Design review of the part built by this model. Coordinates are the model's own, in mm. A direction names the side the tool comes from. Coordinates: 2 decimals unless noted, no trailing zeros. Loops run counter-clockwise (first coordinate to the right, second up) from the corner with the lowest first, then second, coordinate; pieces in that order, holes last. Notation, with made-up numbers: (-31, 34.25) -> (-8, 34.25) arc R19 cw to (-8, 43.25) -> close; hole circle Ø2 at (29, 15). An arc over 180 degrees is marked (long way). Answer in a Markdown table with one row per item.
```python
from build123d import *

# Parameters (mm, degrees)
BOSS_EXTRUDE2_DEPTH = 30
CUT_EXTRUDE3_DEPTH  = 28
SKETCH10_W          = 9
SKETCH10_H          = 11
CUT_EXTRUDE4_DEPTH  = 3


with BuildPart() as part:
    # Sketch2 → Boss-Extrude2 (new body)
    with BuildSketch(Plane.XY):
        with BuildLine():
            Line((-28.917214192, 20.79500657), (39.082785808, 20.79500657))
            ThreePointArc((39.082785808, 20.79500657), (41.204106152, 19.916326914), (42.082785808, 17.79500657))
            Line((42.082785808, 17.79500657), (42.082785808, -56.20499343))
            ThreePointArc((42.082785808, -56.20499343), (41.204106152, -58.326313773), (39.082785808, -59.20499343))
            Line((39.082785808, -59.20499343), (-28.917214192, -59.20499343))
            ThreePointArc((-28.917214192, -59.20499343), (-31.038534535, -58.326313773), (-31.917214192, -56.20499343))
            Line((-31.917214192, -56.20499343), (-31.917214192, 17.79500657))
            ThreePointArc((-31.917214192, 17.79500657), (-31.038534535, 19.916326914), (-28.917214192, 20.79500657))
        make_face()
    extrude(amount=BOSS_EXTRUDE2_DEPTH)

    # Sketch7 → Cut-Extrude3 (cut)
    with BuildSketch(Plane.XY.offset(30)):
        with BuildLine():
            Line((-28.917214192, -57.20499343), (39.082785808, -57.20499343))
            ThreePointArc((39.082785808, -57.20499343), (39.789892589, -56.912100211), (40.082785808, -56.20499343))
            Line((40.082785808, -56.20499343), (40.082785808, 17.79500657))
            ThreePointArc((40.082785808, 17.79500657), (39.789892589, 18.502113351), (39.082785808, 18.79500657))
            Line((39.082785808, 18.79500657), (-28.917214192, 18.79500657))
            ThreePointArc((-28.917214192, 18.79500657), (-29.624320973, 18.502113351), (-29.917214192, 17.79500657))
            Line((-29.917214192, 17.79500657), (-29.917214192, -56.20499343))
            ThreePointArc((-29.917214192, -56.20499343), (-29.624320973, -56.912100211), (-28.917214192, -57.20499343))
        make_face()
    extrude(amount=-CUT_EXTRUDE3_DEPTH, mode=Mode.SUBTRACT)

    # Sketch10 → Cut-Extrude4 (cut)
    with BuildSketch(Plane.XZ.offset(59.20499343)):
        Polygon((-12, 11.6), (-9.001867248, 14.598132752), (-3.001867248, 14.598132752), (0, 11.603739153), (0, 3.6), (-12, 3.6), align=None)
        with Locations((21, 9.1)):
            Rectangle(SKETCH10_W, SKETCH10_H)
    extrude(amount=-CUT_EXTRUDE4_DEPTH, mode=Mode.SUBTRACT)


solid = part.part
```
(1) For pin 1 (0.6 mm diameter, centred on y = -58.5, z = 8, fed in from -X); pin 2 (1 mm diameter, centred on y = -58.5, z = 9, fed in from +X); pin 3 (2 mm diameter, centred on x = 31, y = 12, fed in from +Z), all flat-tipped, find the tip position at first contact; note any pin that passes through.
Evaluation:
| item | result |
|---|---|
| pin 1 | stops at x = -31.16 |
| pin 2 | stops at x = 41.49 |
| pin 3 | stops at z = 2 |
(2) Take a section at A-A on z = 5.25. Give the boundary of the cut face in (x, y) (3 decimals), and give its area (3 significant figures).
Evaluation:
| item | result |
|---|---|
| outline | (-31.917, -56.205) arc R3 ccw to (-28.917, -59.205) -> (-12, -59.205) -> (-12, -57.205) -> (-28.917, -57.205) arc R1 cw to (-29.917, -56.205) -> (-29.917, 17.795) arc R1 cw to (-28.917, 18.795) -> (39.083, 18.795) arc R1 cw to (40.083, 17.795) -> (40.083, -56.205) arc R1 cw to (39.083, -57.205) -> (25.5, -57.205) -> (25.5, -59.205) -> (39.083, -59.205) arc R3 ccw to (42.083, -56.205) -> (42.083, 17.795) arc R3 ccw to (39.083, 20.795) -> (-28.917, 20.795) arc R3 ccw to (-31.917, 17.795) -> close; (0, -59.205) -> (16.5, -59.205) -> (16.5, -57.205) -> (0, -57.205) -> close |
| area | 551 mm² |
(3) Tool access review of faces 4 (the flat face through (6, -19, 0)), 5 (the flat face through (-29.917, -19, 16)), 6 (the flat face through (-10.5, -58.2, 13.1)): name each direction out of +Z, -Z, +X, -X, +Y, -Y from which nothing blocks a thin tool from reaching the whole face with its end or side.
Evaluation:
| item | result |
|---|---|
| face 4 | -Z, +X, -X, +Y, -Y |
| face 5 | +Z |
| face 6 | -Y |
(4) Take a section at B-B on x = -6. Give the boundary of the cut face in (y, z) (3 decimals), and give its area (3 significant figures).
Evaluation:
| item | result |
|---|---|
| outline | (-59.205, 0) -> (20.795, 0) -> (20.795, 30) -> (18.795, 30) -> (18.795, 2) -> (-57.205, 2) -> (-57.205, 3.6) -> (-59.205, 3.6) -> close; (-59.205, 14.598) -> (-57.205, 14.598) -> (-57.205, 30) -> (-59.205, 30) -> close |
| area | 250 mm² |
(5) Draft analysis for pull direction X (two halves, no side actions). For faces 1 (the flat face through (5, -19, 2)), 2 (the flat face through (41, -19, 30)), 3 (the flat face through (42.083, -19, 15)), state which applies: pulls with the +X half, pulls with the -X half, needs draft (parallel to the pull), parting line crosses it, or undercut.
Evaluation:
| item | result |
|---|---|
| face 1 | undercut |
| face 2 | needs draft |
| face 3 | pulls with the +X half |
(6) Take a section at D-D on y = -42.5. Give the boundary of the cut face in (x, z), and give its area (3 significant figures).
Evaluation:
| item | result |
|---|---|
| outline | (-31.92, 0) -> (42.08, 0) -> (42.08, 30) -> (40.08, 30) -> (40.08, 2) -> (-29.92, 2) -> (-29.92, 30) -> (-31.92, 30) -> close |
| area | 260 mm² |
(7) To check wall thickness, follow probe 1 along X at (y, z) = (-18, 23.5); probe 2 along Y at (x, z) = (-20, 13.25) (3 decimals); probe 3 along Z at (x, y) = (-2, -16). State the ranges of each line that lie inside material, in increasing order.
Evaluation:
| item | result |
|---|---|
| probe 1 | x = -31.92 to -29.92, 40.08 to 42.08 |
| probe 2 | y = -59.205 to -57.205, 18.795 to 20.795 |
| probe 3 | z = 0 to 2 |
(8) Take a section at C-C on z = 18.25. Give the boundary of the cut face in (x, y) (3 decimals), and give its area (3 significant figures).
Evaluation:
| item | result |
|---|---|
| outline | (-31.917, -56.205) arc R3 ccw to (-28.917, -59.205) -> (39.083, -59.205) arc R3 ccw to (42.083, -56.205) -> (42.083, 17.795) arc R3 ccw to (39.083, 20.795) -> (-28.917, 20.795) arc R3 ccw to (-31.917, 17.795) -> close; hole (-29.917, -56.205) arc R1 ccw to (-28.917, -57.205) -> (39.083, -57.205) arc R1 ccw to (40.083, -56.205) -> (40.083, 17.795) arc R1 ccw to (39.083, 18.795) -> (-28.917, 18.795) arc R1 ccw to (-29.917, 17.795) -> close |
| area | 593 mm² |
